```python
from build123d import *

# Parameters (mm, degrees)
EXTRUDE_1_DEPTH      = 3
SKETCH_2_R           = 1.5
CUT_EXTRUDE_7_DEPTH  = 43.02014847
SKETCH_4_R           = 1.5
CUT_EXTRUDE_8_DEPTH  = 43.02014847
SKETCH_5_R           = 3.01
CUT_EXTRUDE_9_DEPTH  = 43.02014847
SKETCH_6_R           = 1.5
CUT_EXTRUDE_10_DEPTH = 43.02014847


with BuildPart() as part:
    # 草图1 → 凸台-拉伸1 (new body)
    with BuildSketch(Plane.XY):
        Polygon((-7.5, 0), (7.5, 0), (7.5, 5.665837688), (17.5, 5.665837688), (30, -1.269316313), (30, -29.269316313), (-30, -29.269316313), (-30, -1.269316313), (-17.5, 5.665837688), (-7.5, 5.665837688), align=None)
    extrude(amount=EXTRUDE_1_DEPTH)

    # 草图2 → 切除-拉伸7 (cut, through all)
    with BuildSketch(Plane(origin=(0, 0, 0), x_dir=(-1, 0, 0), z_dir=(0, 0, -1))):
        with Locations((-25.62844718, -17.669380188)):
            Circle(SKETCH_2_R)
        with Locations((-25.62844718, -7.669380188)):
            Circle(SKETCH_2_R)
        with Locations((23.37155282, -17.669380188)):
            Circle(SKETCH_2_R)
        with Locations((23.37155282, -7.669380188)):
            Circle(SKETCH_2_R)
    extrude(amount=-CUT_EXTRUDE_7_DEPTH, mode=Mode.SUBTRACT)

    # 草图4 → 切除-拉伸8 (cut, through all)
    with BuildSketch(Plane(origin=(0, 0, 0), x_dir=(-1, 0, 0), z_dir=(0, 0, -1))):
        with Locations((-11.696832964, 2.350343297)):
            Circle(SKETCH_4_R)
        with Locations((11.682164636, 2.350343297)):
            Circle(SKETCH_4_R)
    extrude(amount=-CUT_EXTRUDE_8_DEPTH, mode=Mode.SUBTRACT)

    # 草图5 → 切除-拉伸9 (cut, through all)
    with BuildSketch(Plane(origin=(0, 0, 0), x_dir=(-1, 0, 0), z_dir=(0, 0, -1))):
        with Locations((10.34155282, -12.669316313)):
            Circle(SKETCH_5_R)
        with Locations((-12.15844718, -12.669380188)):
            Circle(SKETCH_5_R)
    extrude(amount=-CUT_EXTRUDE_9_DEPTH, mode=Mode.SUBTRACT)

    # 草图6 → 切除-拉伸10 (cut, through all)
    with BuildSketch(Plane(origin=(0, 0, 0), x_dir=(-1, 0, 0), z_dir=(0, 0, -1))):
        with Locations((14, -26.769316313)):
            Circle(SKETCH_6_R)
        with Locations((-14, -26.769316313)):
            Circle(SKETCH_6_R)
    extrude(amount=-CUT_EXTRUDE_10_DEPTH, mode=Mode.SUBTRACT)


solid = part.part
```
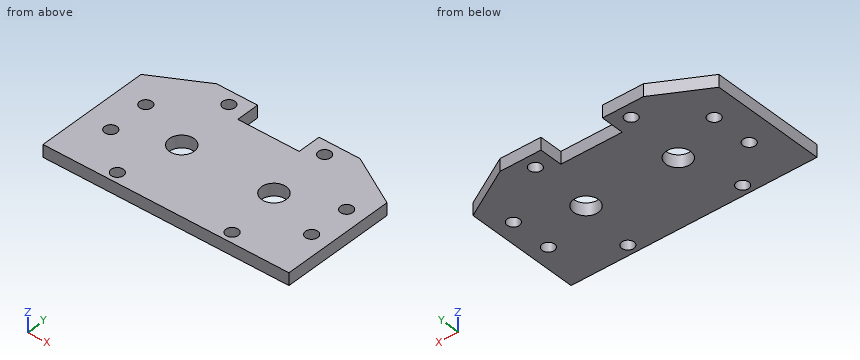
Here's how the part is built. I have some questions about the finished solid (model axes, mm). Coordinates: 2 decimals unless noted, no trailing zeros. Loops run counter-clockwise (first coordinate to the right, second up) from the corner with the lowest first, then second, coordinate; pieces in that order, holes last. Notation, with made-up numbers: M -15.5,70.25 L 19.5,70.25 A13 ccw 19.5,86.25 Z; hole C 5,13.5 d11. An arc over 180 degrees is marked long. One line per item, written item: value.
1. Imagine slicing it at D-D (z = 1.85). State how many separate pieces and enclosed holes the cut face has, and give its area (3 significant figures).
Geometry says:
separate pieces: 1
enclosed holes: 10
area: 1,810 mm2
2. Will these pins go through, and if not, where does the flat tip stop? pin 1 Ø2.5 at (x, y) = (-23.37, -17.67) entering from -Z; pin 2 Ø1.5 at (x, z) = (-2.5, 1) entering from +Y.
Geometry says:
pin 1: passes through
pin 2: stops at y = 0
3. Imagine slicing it at A-A (x = -14). List the corners of the cut face in (y, z) for me, and give its area (3 significant figures).
Geometry says:
outline: M -29.27,0 L -28.27,0 L -28.27,3 L -29.27,3 Z; M -25.27,0 L 5.67,0 L 5.67,3 L -25.27,3 Z
area: 95.8 mm2
4. Please list where these lines run through material, in increasing order: probe 1 along Y at (x, z) = (14.5, 2.05); probe 2 along X at (y, z) = (-26.5, 1.3); probe 3 along Y at (x, z) = (-23.5, 2.3).
Geometry says:
probe 1: y = -29.27 to -28.18, -25.36 to -14.56, -10.78 to 5.67
probe 2: x = -30 to -15.48, -12.52 to 12.52, 15.48 to 30
probe 3: y = -29.27 to -19.16, -16.17 to -9.16, -6.17 to 2.34
5. Imagine slicing it at B-B (x = -23). List the corners of the cut face in (y, z) for me, and give its area (3 significant figures).
Geometry says:
outline: M -29.27,0 L -19.12,0 L -19.12,3 L -29.27,3 Z; M -16.22,0 L -9.12,0 L -9.12,3 L -16.22,3 Z; M -6.22,0 L 2.61,0 L 2.61,3 L -6.22,3 Z
area: 78.2 mm2
6. Imagine slicing it at C-C (y = -12). List the corners of the cut face in (x, z) for me, and give its area (3 significant figures).
Geometry says:
outline: M -30,0 L -13.28,0 L -13.28,3 L -30,3 Z; M -7.41,0 L 9.22,0 L 9.22,3 L -7.41,3 Z; M 15.09,0 L 30,0 L 30,3 L 15.09,3 Z
area: 145 mm2
